from build123d import *

# Parameters (mm, degrees)
SKETCH_R    = 4
SKETCH_R_2  = 1.6
PAD_DEPTH   = 3
FILLET_R    = 25
FILLET012_R = 37


with BuildPart() as part:
    # Sketch → Pad (new body)
    with BuildSketch(Plane.YZ):
        with BuildLine():
            ThreePointArc((0, 8), (-7.980512, 0.558052), (-1.113385, -7.922145))
            Line((-1.113385, -7.922145), (18.3, -10.650518))
            Line((27.656685, -63.714914), (18.3, -10.650518))
            ThreePointArc((27.656685, -63.714914), (36.924332, -70.20419), (43.413609, -60.936543))
            Line((31.258236, 8), (43.413609, -60.936543))
            Line((0, 8), (31.258236, 8))
        make_face()
        Circle(SKETCH_R, mode=Mode.SUBTRACT)
        with Locations((32.383762, -62.881402)):
            Circle(SKETCH_R_2, mode=Mode.SUBTRACT)
        with Locations((38.686532, -61.770054)):
            Circle(SKETCH_R_2, mode=Mode.SUBTRACT)
    extrude(amount=PAD_DEPTH)

    # Fillet
    fillet_edges = [part.edges().sort_by_distance(p)[0] for p in [
        (1.5, 18.3, -10.650518),
    ]]
    fillet(fillet_edges, radius=FILLET_R)

    # Fillet012
    fillet012_edges = [part.edges().sort_by_distance(p)[0] for p in [
        (1.5, 31.258236, 8),
    ]]
    fillet(fillet012_edges, radius=FILLET012_R)


with BuildPart() as part_1:
    # Body placement: moved
    add(part.part.moved(Location((44, 0, 0))))


solid = part_1.part
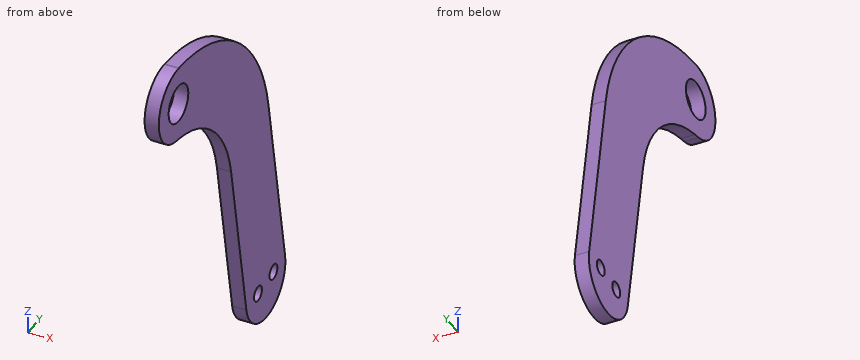
The listing builds one solid part. Answer for the finished solid, in the listing's coordinates (mm). Round coordinates to 2 decimals unless told otherwise and drop trailing zeros. Write each loop counter-clockwise with the first axis right and the second up, starting at its lowest first coordinate (ties: lowest second). Pieces come first, ordered by that corner, then holes. Notation, with made-up numbers: M -14,-35.75 L 44,-35.75 A13 cw 44,-25.75 Z; hole C 39,30 d7. An arc over 180 degrees is marked long. Write each question's results on one line, items separated by ' | '. Start each with the question number.
(1) The part is cut by section A-A, the plane z = 0. Write down the section's boundary in (x, y).
(2) The part is cut by section B-B, the plane y = 33. Write down the section's boundary in (x, z).
(3) Find the intervals of material crossed by line 1 (Z direction, x = 45.4, y = 0); line 2 (Z direction, x = 45.85, y = -1); line 3 (Y direction, x = 46.15, z = 1), in increasing order.
(4) The part is cut by section C-C, the plane x = 46.4. Write down the section's boundary in (y, z).
(5) The part is cut by section D-D, the plane z = -48.5. Write down the section's boundary in (x, y), and give its area (3 significant figures).
Worked answers:
1) outline: M 44,-8 L 47,-8 L 47,-4 L 44,-4 Z; M 44,4 L 47,4 L 47,23.19 L 44,23.19 Z
2) outline: M 44,-69.91 L 47,-69.91 L 47,-64.36 L 44,-64.36 Z; M 44,-61.4 L 47,-61.4 L 47,-11.86 L 44,-11.86 Z
3) line 1: z = -8.08 to -4, 4 to 8 | line 2: z = -7.94 to -3.87, 3.87 to 7.94 | line 3: y = -7.94 to -3.87, 3.87 to 21.87
4) outline: M -1.11,-7.92 L 0.31,-8.12 A25 cw 21.45,-28.54 L 27.66,-63.71 A8 ccw 43.41,-60.94 L 36.65,-22.58 A37 ccw 0.21,8 L 0,8 A8 ccw Z; hole C 0,0 d8; hole C 32.38,-62.88 d3.2; hole C 38.69,-61.77 d3.2
5) outline: M 44,24.97 L 47,24.97 L 47,41.22 L 44,41.22 Z | area: 48.7 mm²
